Read the model definition and answer for the solid it produces. Units are mm, in the model's axes. A direction names the side the tool comes from. Coordinates: 2 decimals unless noted, no trailing zeros. Write each loop counter-clockwise with the first axis right and the second up, starting at its lowest first coordinate (ties: lowest second). Pieces come first, ordered by that corner, then holes. Notation, with made-up numbers: (69, 49) -> (114, 49) arc R17 cw to (114, 80) -> close; hole circle Ø5 at (22, 43). An arc over 180 degrees is marked (long way). Return JSON: item names as keys, results as strings.
from build123d import *

# Parameters (mm, degrees)
SKETCH_W      = 110
SKETCH_H      = 20
PAD_DEPTH     = 3
SKETCH001_W   = 110
SKETCH001_H   = 5
PAD001_DEPTH  = 3
SKETCH002_W   = 110
SKETCH002_H   = 20
SKETCH002_W_2 = 95.5
SKETCH002_H_2 = 3
PAD002_DEPTH  = 3


with BuildPart() as part:
    # Sketch → Pad (new body)
    with BuildSketch(Plane.XY):
        Rectangle(SKETCH_W, SKETCH_H)
    extrude(amount=PAD_DEPTH)

    # Sketch001 (on Face6 of Pad) → Pad001 (join)
    with BuildSketch(Plane.XY.offset(3)):
        with Locations((0, 7.5)):
            Rectangle(SKETCH001_W, SKETCH001_H)
        with Locations((0, -7.5)):
            Rectangle(SKETCH001_W, SKETCH001_H)
    extrude(amount=PAD001_DEPTH)

    # Sketch002 (on Face12 of Pad001) → Pad002 (join)
    with BuildSketch(Plane.XY.offset(6)):
        Rectangle(SKETCH002_W, SKETCH002_H)
        Rectangle(SKETCH002_W_2, SKETCH002_H_2, mode=Mode.SUBTRACT)
    extrude(amount=PAD002_DEPTH)


solid = part.part
1. For a pull along Z with two mould halves and no side action, classify faces 1 (the face through (47.75, 0, 7)), 2 (the face through (-1, -5, 4)), 3 (the face through (-1, 0, 0)) as +Z half, -Z half, draft (parallel to the pull), parting line (faces both ways), or undercut.
Taken from the geometry:
{"face 1": "draft", "face 2": "undercut", "face 3": "-Z half"}
2. The part is cut by section A-A (z = 8). Determine the outline of the cut face in (x, y), then the cut area to 3 significant figures.
Taken from the geometry:
{"outline": "(-55, -10) -> (55, -10) -> (55, 10) -> (-55, 10) -> close; hole (-47.75, -1.5) -> (47.75, -1.5) -> (47.75, 1.5) -> (-47.75, 1.5) -> close", "area": "1,910 mm2"}
3. The part is cut by section B-B (y = -4). Determine the outline of the cut face in (x, z).
Taken from the geometry:
{"outline": "(-55, 0) -> (55, 0) -> (55, 3) -> (-55, 3) -> close; (-55, 6) -> (55, 6) -> (55, 9) -> (-55, 9) -> close"}
4. Consider L1, parallel to Y at x = -36, z = 7; L2, parallel to Z at x = -33, y = 4.5; L3, parallel to X at y = 1.25, z = 7. Determine where each line is inside the solid, lowest interval first.
Taken from the geometry:
{"L1": "y = -10 to -1.5, 1.5 to 10", "L2": "z = 0 to 3, 6 to 9", "L3": "x = -55 to -47.75, 47.75 to 55"}
5. A tool of negligible diameter and unlimited length cuts with its end or side. For faces 4 (the face through (-1, -2, 9)), 5 (the face through (-1, 1.5, 7)), 6 (the face through (-1, 5, 4)), from which of +Z, -Z, +X, -X, +Y, -Y can it reach the whole face along a straight path? Write none if from no direction.
Taken from the geometry:
{"face 4": "+Z, +X, -X, +Y, -Y", "face 5": "+Z", "face 6": "+X, -X"}
6. The part is cut by section C-C (x = -3.5). Determine the outline of the cut face in (y, z).
Taken from the geometry:
{"outline": "(-10, 0) -> (10, 0) -> (10, 9) -> (1.5, 9) -> (1.5, 6) -> (5, 6) -> (5, 3) -> (-5, 3) -> (-5, 6) -> (-1.5, 6) -> (-1.5, 9) -> (-10, 9) -> close"}
